from build123d import *

# Parameters (mm, degrees)
BOSS_EXTRUDE1_DEPTH = 3.175
SKETCH3_W           = 3.5
SKETCH3_H           = 10
CUT_EXTRUDE1_DEPTH  = 4.175


with BuildPart() as part:
    # Sketch2 → Boss-Extrude1 (new body)
    with BuildSketch(Plane(origin=(0, 0, 0), x_dir=(1, 0, 0), z_dir=(0, 1, 0))):
        Polygon((0, 0), (-5, 0), (-65, 85), (-45, 85), (0, 20), (200, 20), (245, 85), (265, 85), (205, 0), (200, 0), align=None)
    extrude(amount=BOSS_EXTRUDE1_DEPTH)

    # Sketch3 → Cut-Extrude1 (cut, through all)
    with BuildSketch(Plane(origin=(0, 3.175, 0), x_dir=(1, 0, 0), z_dir=(0, 1, 0))):
        with Locations((41.05, 15)):
            Rectangle(SKETCH3_W, SKETCH3_H)
        with Locations((1.75, 15)):
            Rectangle(SKETCH3_W, SKETCH3_H)
        with Locations((80.35, 15)):
            Rectangle(SKETCH3_W, SKETCH3_H)
        with Locations((119.65, 15)):
            Rectangle(SKETCH3_W, SKETCH3_H)
        with Locations((158.95, 15)):
            Rectangle(SKETCH3_W, SKETCH3_H)
        with Locations((198.25, 15)):
            Rectangle(SKETCH3_W, SKETCH3_H)
    extrude(amount=-CUT_EXTRUDE1_DEPTH, mode=Mode.SUBTRACT)


solid = part.part
Can you work these out from the model? Positions are in its coordinate system, mm. Give positions to 0.01 mm unless a question says otherwise; leave off trailing zeros. Order: outer loops, then holes, each group sorted by start corner. A loop starts at its lowest first (then second) coordinate and runs counter-clockwise, first axis right, second up. Notation, with made-up numbers: M -12.75,14 L 15.25,14 A25 cw 15.25,40 Z; hole C 85,18.25 d8. An arc over 180 degrees is marked long. One line per item, written item: value.
Item 1: If we section it at A-A on z = -23: Write out the boundary of the cut face in (x, y) (3 decimals).
Verdict:
outline: M -21.235,0 L -2.077,0 L -2.077,3.175 L -21.235,3.175 Z; M 202.077,0 L 221.235,0 L 221.235,3.175 L 202.077,3.175 Z
Item 2: If we mould it in two halves opening along X, with no side actions, what happens to faces 1 (the face through (222.185, 1.565, -52.045)), 2 (the face through (101, 3.175, -18)), 3 (the face through (235.42, 1.565, -43.095)), 4 (the face through (-22.81, 1.57, -52.95))? For each: pulls with the +X half, pulls with the -X half, needs draft (parallel to the pull), parting line crosses it, or undercut.
Verdict:
face 1: undercut
face 2: needs draft
face 3: pulls with the +X half
face 4: undercut
Item 3: If we section it at C-C on z = -71: Write out the boundary of the cut face in (x, y) (3 decimals), and give its area (3 significant figures).
Verdict:
outline: M -55.118,0 L -35.308,0 L -35.308,3.175 L -55.118,3.175 Z; M 235.308,0 L 255.118,0 L 255.118,3.175 L 235.308,3.175 Z
area: 126 mm2
Item 4: For pin 1 (1.6 mm diameter, centred on y = 2, z = -17, fed in from +X); pin 2 (1.6 mm diameter, centred on x = 134, y = 1, fed in from -Z); pin 3 (1.6 mm diameter, centred on y = 2, z = -15, fed in from -X), each with a flat end and sliding along its axis, tell me the tip position at first contact or that it passes through.
Verdict:
pin 1: x = 217.56
pin 2: z = -20
pin 3: x = -16.15
Item 5: Please list where these lines run through material, in increasing order: line 1 (X direction, y = 0.6, z = -55.5); line 2 (X direction, y = 2.4, z = -60); line 3 (Z direction, x = 167, y = 3.05).
Verdict:
line 1: -44.18 to -24.58, 224.58 to 244.18
line 2: -47.35 to -27.69, 227.69 to 247.35
line 3: -20 to 0
Item 6: If we section it at D-D on x = 51: Write out the boundary of the cut face in (y, z) (3 decimals), and give its area (3 significant figures).
Verdict:
outline: M 0,-20 L 3.175,-20 L 3.175,0 L 0,0 Z
area: 63.5 mm2
